```python
from build123d import *

# Parameters (mm, degrees)
SKETCH1_W           = 60
SKETCH1_H           = 45
BOSS_EXTRUDE1_DEPTH = 10
SKETCH2_W           = 70
SKETCH2_H           = 18
BOSS_EXTRUDE2_DEPTH = 7.5
CUT_EXTRUDE1_DEPTH  = 5
SKETCH4_W           = 4.5
SKETCH4_H           = 4
BOSS_EXTRUDE3_DEPTH = 2
SKETCH5_R           = 1.5
CUT_EXTRUDE2_DEPTH  = 15


with BuildPart() as part:
    # Sketch1 → Boss-Extrude1 (new body)
    with BuildSketch(Plane(origin=(0, 0, 0), x_dir=(1, 0, 0), z_dir=(0, 1, 0))):
        Rectangle(SKETCH1_W, SKETCH1_H)
    extrude(amount=BOSS_EXTRUDE1_DEPTH)

    # Sketch2 → Boss-Extrude2 (add)
    with BuildSketch(Plane.XY.offset(22.5)):
        with Locations((0, 5)):
            Rectangle(SKETCH2_W, SKETCH2_H)
    extrude(amount=BOSS_EXTRUDE2_DEPTH)

    # Sketch3 → Cut-Extrude1 (cut)
    with BuildSketch(Plane(origin=(0, 10, 0), x_dir=(1, 0, 0), z_dir=(0, 1, 0))):
        with BuildLine():
            ThreePointArc((-19.5325, -13.495), (-18.170661955, -18.166166123), (-13.49, -19.495))
            add(Edge.make_bspline(
                [(-13.49, -19.495), (-4.496666667, -17.441666667), (4.496666667, -17.441666667), (13.49, -19.495)],
                knots=[0, 0, 0, 0, 1, 1, 1, 1], degree=3))
            ThreePointArc((13.49, -19.495), (18.162524477, -18.157971004), (19.5325, -13.495))
            add(Edge.make_bspline(
                [(19.5325, 13.495), (16.4925, 0), (19.5325, -13.495)],
                knots=[0, 0, 0, 1, 1, 1], degree=2))
            ThreePointArc((19.5325, 13.495), (18.162524477, 18.157971004), (13.49, 19.495))
            add(Edge.make_bspline(
                [(-13.49, 19.495), (-4.496666667, 17.441666667), (4.496666667, 17.441666667), (13.49, 19.495)],
                knots=[0, 0, 0, 0, 1, 1, 1, 1], degree=3))
            ThreePointArc((-13.49, 19.495), (-18.170661955, 18.166166123), (-19.5325, 13.495))
            add(Edge.make_bspline(
                [(-19.5325, 13.495), (-18.519166667, 8.996666667), (-17.505833333, 0), (-18.519166667, -8.996666667), (-19.5325, -13.495)],
                knots=[0, 0, 0, 0, 0.5, 1, 1, 1, 1], degree=3))
        make_face()
    extrude(amount=-CUT_EXTRUDE1_DEPTH, mode=Mode.SUBTRACT)

    # Sketch4 → Boss-Extrude3 (add)
    with BuildSketch(Plane(origin=(35, 0, 0), x_dir=(0, 0, -1), z_dir=(1, 0, 0))):
        Polygon((-30, 5), (-30, 8.2), (-10, 8.2), (-10, 1.8), (-30, 1.8), align=None)
        with Locations((-14.75, 5)):
            Rectangle(SKETCH4_W, SKETCH4_H, mode=Mode.SUBTRACT)
    boss_extrude3 = extrude(amount=BOSS_EXTRUDE3_DEPTH)

    # Mirror1: Boss-Extrude3 across plane
    add(boss_extrude3.mirror(Plane(origin=(0, 0, 0), x_dir=(0, 0, 1), z_dir=(1, 0, 0))))

    # Sketch5 → Cut-Extrude2 (cut, through all)
    with BuildSketch(Plane(origin=(0, 10, 0), x_dir=(1, 0, 0), z_dir=(0, 1, 0))):
        with Locations((25.5, 12.5)):
            Circle(SKETCH5_R)
    cut_extrude2 = extrude(amount=-CUT_EXTRUDE2_DEPTH, mode=Mode.SUBTRACT)

    # Mirror2: Cut-Extrude2 across plane
    add(cut_extrude2.mirror(Plane(origin=(0, 0, 0), x_dir=(0, 0, 1), z_dir=(1, 0, 0))), mode=Mode.SUBTRACT)


solid = part.part
```
Part model, mm, in its own coordinate system. A direction names the side the tool comes from. Give positions to 0.01 mm unless a question says otherwise; leave off trailing zeros. Order: outer loops, then holes, each group sorted by start corner. A loop starts at its lowest first (then second) coordinate and runs counter-clockwise, first axis right, second up. Notation, with made-up numbers: M 58.25,67.5 L 70.25,67.5 A21 cw 70.25,106.5 Z; hole C 20,23.5 d3. An arc over 180 degrees is marked long. Use a Markdown table: item, result. Add a question column.
(1) 3-axis set-ups, long thin cutter, end or side, ignore diameter. For faces 1 (the face through (-18.221, 7.535, 18.116)), 2 (the face through (35, -1, 26)), 3 (the face through (-36, 5, 17)), 4 (the face through (-36, 8.2, 20)): which of +Z, -Z, +X, -X, +Y, -Y reach the whole face in a straight line?
(2) Saw through at C-C, the plane y = -1. Give the cut face in (x, z), and give its area (3 significant figures).
(3) Saw through at A-A, the plane x = -25.5. Give the cut face in (y, z), and give its area (3 significant figures).
(4) Probe line 1 along X through (y, z) = (3.25, -12.5); line 2 along X through (y, z) = (8, 21.5); line 3 along X through (y, z) = (6.75, -12.5). List the from-to ranges inside material, lowest first. Write a range as [from, to].
(5) Mould opens along Z. For faces 5 (the face through (36, 3, 15)), 6 (the face through (-30, 5, 0)), 7 (the face through (36, 5, 10)) say: +Z half, -Z half, draft (parallel to the pull), parting line (faces both ways), or undercut.
(6) Saw through at D-D, the plane z = -12.5. Give the number of separate pieces and of enclosed holes in the cut face, and give its area (3 significant figures).
(7) Saw through at B-B, the plane z = 24. Give the cut face in (x, y), and give its area (3 significant figures).
(8) Drop flat-ended pins along their axis: P1, Ø2, axis at x = 24.5, z = 3.5, coming from the -Y side; P2, Ø6, axis at y = -2, z = 24.5, coming from the +X side; P3, Ø0.6, axis at x = -35.5, z = 13.5, coming from the +Y side. Give the stop position or say it passes through.
Answer key:
| question | item | result |
|---|---|---|
| 1 | face 1 | +Y |
| 1 | face 2 | +Z, -Z, +X, -Y |
| 1 | face 3 | -X |
| 1 | face 4 | +Z, -Z, -X, +Y |
| 2 | outline | M -35,22.5 L 35,22.5 L 35,30 L -35,30 Z |
| 2 | area | 525 mm^2 |
| 3 | outline | M -4,22.5 L 0,22.5 L 0,-11 L 10,-11 L 10,22.5 L 14,22.5 L 14,30 L -4,30 Z; M 0,-22.5 L 10,-22.5 L 10,-14 L 0,-14 Z |
| 3 | area | 555 mm^2 |
| 4 | line 1 | [-30, -27], [-24, 24], [27, 30] |
| 4 | line 2 | [-37, -35], [-30, 30], [35, 37] |
| 4 | line 3 | [-30, -27], [-24, -19.32], [19.32, 24], [27, 30] |
| 5 | face 5 | undercut |
| 5 | face 6 | draft |
| 5 | face 7 | -Z half |
| 6 | separate pieces | 3 |
| 6 | enclosed holes | 0 |
| 6 | area | 347 mm^2 |
| 7 | outline | M -37,1.8 L -35,1.8 L -35,-4 L 35,-4 L 35,1.8 L 37,1.8 L 37,8.2 L 35,8.2 L 35,14 L -35,14 L -35,8.2 L -37,8.2 Z |
| 7 | area | 1,290 mm^2 |
| 8 | P1 | y = 0 |
| 8 | P2 | x = 35 |
| 8 | P3 | y = 8.2 |
